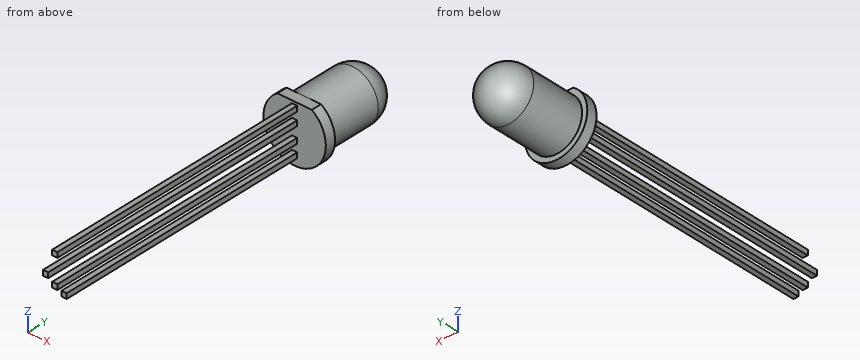
from build123d import *

# Parameters (mm, degrees)
CUT_EXTRUDE2_DEPTH      = 10
SKETCH3_W               = 0.5
SKETCH3_H               = 0.5
BOSS_EXTRUDE1_DEPTH     = 27
SKETCH5_W               = 0.5
SKETCH5_H               = 1
CUT_EXTRUDE3_DEPTH      = 4
CUT_EXTRUDE3_DEPTH_BACK = 4
SKETCH7_W               = 0.5
SKETCH7_H               = 2
CUT_EXTRUDE4_DEPTH      = 4
CUT_EXTRUDE4_DEPTH_BACK = 4


with BuildPart() as part:
    # Sketch1 → Revolve1 (revolve)
    with BuildSketch(Plane(origin=(0, 0, 0), x_dir=(0, 0, -1), z_dir=(1, 0, 0))):
        with BuildLine():
            Line((0, 0), (3, 0))
            Line((3, 0), (3, 1))
            Line((3, 1), (2.5, 1))
            Line((2.5, 1), (2.5, 6.25))
            ThreePointArc((2.5, 6.25), (1.767766953, 8.017766953), (0, 8.75))
            Line((0, 8.75), (0, 0))
        make_face()
    revolve(axis=Axis((0, 8.75, 0), (0, -1, 0)))

    # Sketch2 → Cut-Extrude2 (cut)
    with BuildSketch(Plane(origin=(0, 0, 0), x_dir=(1, 0, 0), z_dir=(0, 1, 0))):
        with BuildLine():
            Line((-1.658312395, -2.5), (1.658312395, -2.5))
            ThreePointArc((1.658312395, -2.5), (0, -3), (-1.658312395, -2.5))
        make_face()
    extrude(amount=CUT_EXTRUDE2_DEPTH, mode=Mode.SUBTRACT)

    # Sketch3 → Boss-Extrude1 (add)
    with BuildSketch(Plane.XZ):
        with Locations((0, 2)):
            Rectangle(SKETCH3_W, SKETCH3_H)
        with Locations((0, 0.75)):
            Rectangle(SKETCH3_W, SKETCH3_H)
        with Locations((0, -0.75)):
            Rectangle(SKETCH3_W, SKETCH3_H)
        with Locations((0, -2)):
            Rectangle(SKETCH3_W, SKETCH3_H)
    extrude(amount=BOSS_EXTRUDE1_DEPTH)

    # Sketch5 → Cut-Extrude3 (cut, two sides)
    with BuildSketch(Plane(origin=(0, 0, 0), x_dir=(0, 0, -1), z_dir=(1, 0, 0))) as cut_extrude3_sk:
        with Locations((-2, -26.5)):
            Rectangle(SKETCH5_W, SKETCH5_H)
        with Locations((0.75, -26.5)):
            Rectangle(SKETCH5_W, SKETCH5_H)
    extrude(amount=CUT_EXTRUDE3_DEPTH, mode=Mode.SUBTRACT)
    extrude(cut_extrude3_sk.sketch, amount=-CUT_EXTRUDE3_DEPTH_BACK, mode=Mode.SUBTRACT)

    # Sketch7 → Cut-Extrude4 (cut, two sides)
    with BuildSketch(Plane(origin=(0, 0, 0), x_dir=(0, 0, -1), z_dir=(1, 0, 0))) as cut_extrude4_sk:
        with Locations((2, -26)):
            Rectangle(SKETCH7_W, SKETCH7_H)
    extrude(amount=CUT_EXTRUDE4_DEPTH, mode=Mode.SUBTRACT)
    extrude(cut_extrude4_sk.sketch, amount=-CUT_EXTRUDE4_DEPTH_BACK, mode=Mode.SUBTRACT)


solid = part.part
Could you check a few things on this model? Use its own coordinates, in mm. Coordinates: 2 decimals unless noted, no trailing zeros. Order: outer loops, then holes, each group sorted by start corner. A loop starts at its lowest first (then second) coordinate and runs counter-clockwise, first axis right, second up. Notation, with made-up numbers: (16.5, 61) - (21.5, 61) arc R34 cw to (21.5, 100) - close; hole circle Ø2 at (84.5, 32.25). An arc over 180 degrees is marked (long way). Answer in a Markdown table with one row per item. Add a question column.
(1) If we section it at C-C, the plane x = 1.15: Please give me the cut outline in (y, z).
(2) Will these pins go through, and if not, where does the flat tip stop? pin 1 (2 mm diameter, centred on x = -1.5, z = -2, fed in from -Y); pin 2 (0.6 mm diameter, centred on x = 0, z = 2, fed in from -Y); pin 3 (2 mm diameter, centred on y = -16.5, z = 2, fed in from +X).
(3) If we section it at A-A, the plane y = -3.5: Please give me the cut outline in (x, z), then the cut area to 3 significant figures.
(4) If we section it at B-B, the plane z = 0: Please give me the cut outline in (x, y), then the cut area to 3 significant figures.
(5) I need wall thicknesses on L1, parallel to X at y = -4, z = 0.85; L2, parallel to Z at x = 0.2, y = 5; L3, parallel to Y at x = 1.4, z = 0.05. Which ranges of each line are inside material? Lowest first, please.
Results are:
| question | item | result |
|---|---|---|
| 1 | outline | (0, -2.77) - (1, -2.77) - (1, -2.22) - (6.25, -2.22) arc R2.22 ccw to (6.25, 2.22) - (1, 2.22) - (1, 2.5) - (0, 2.5) - close |
| 2 | pin 1 | stops at y = 0 |
| 2 | pin 2 | stops at y = -26 |
| 2 | pin 3 | stops at x = 0.25 |
| 3 | outline | (-0.25, -2.25) - (0.25, -2.25) - (0.25, -1.75) - (-0.25, -1.75) - close; (-0.25, -1) - (0.25, -1) - (0.25, -0.5) - (-0.25, -0.5) - close; (-0.25, 0.5) - (0.25, 0.5) - (0.25, 1) - (-0.25, 1) - close; (-0.25, 1.75) - (0.25, 1.75) - (0.25, 2.25) - (-0.25, 2.25) - close |
| 3 | area | 1.00 mm2 |
| 4 | outline | (-3, 0) - (3, 0) - (3, 1) - (2.5, 1) - (2.5, 6.25) arc R2.5 ccw to (-2.5, 6.25) - (-2.5, 1) - (-3, 1) - close |
| 4 | area | 42.1 mm2 |
| 5 | L1 | x = -0.25 to 0.25 |
| 5 | L2 | z = -2.49 to 2.49 |
| 5 | L3 | y = 0 to 8.32 |
